For this review, take the finished solid that the model builds, in its own axes (mm). A direction names the side the tool comes from. Round coordinates to 2 decimals unless told otherwise and drop trailing zeros. Loops run counter-clockwise (first coordinate to the right, second up) from the corner with the lowest first, then second, coordinate; pieces in that order, holes last. Notation, with made-up numbers: (85.5, 28) -> (104.5, 28) arc R15 ccw to (104.5, 35) -> close; hole circle Ø3 at (80.5, 89). An arc over 180 degrees is marked (long way). Write each question's results on one line, items separated by ' | '.
```python
from build123d import *

# Parameters (mm, degrees)
SKETCH011_W             = 2000
SKETCH011_H             = 1000
PAD004_DEPTH            = 50
SKETCH012_W             = 100
SKETCH012_H             = 100
PAD005_DEPTH            = 900
SKETCH013_W             = 100
SKETCH013_H             = 100
PAD006_DEPTH            = 900
SKETCH014_W             = 100
SKETCH014_H             = 100
PAD007_DEPTH            = 900
SKETCH015_W             = 100
SKETCH015_H             = 100
PAD008_DEPTH            = 900
FILLET010_R             = 45
BODY002_PLACEMENT_ANGLE = 90


with BuildPart() as part:
    # Sketch011 → Pad004 (new body)
    with BuildSketch(Plane.XY):
        with Locations((1000, 500)):
            Rectangle(SKETCH011_W, SKETCH011_H)
    extrude(amount=PAD004_DEPTH)

    # Sketch012 (on Face5 of Pad004) → Pad005 (join)
    with BuildSketch(Plane(origin=(0, 0, 0), x_dir=(1, 0, 0), z_dir=(0, 0, -1))):
        with Locations((200, -200)):
            Rectangle(SKETCH012_W, SKETCH012_H)
    extrude(amount=PAD005_DEPTH)

    # Sketch013 (on Face4 of Pad005) → Pad006 (join)
    with BuildSketch(Plane(origin=(0, 0, 0), x_dir=(1, 0, 0), z_dir=(0, 0, -1))):
        with Locations((1800, -200)):
            Rectangle(SKETCH013_W, SKETCH013_H)
    extrude(amount=PAD006_DEPTH)

    # Sketch014 (on Face4 of Pad006) → Pad007 (join)
    with BuildSketch(Plane(origin=(0, 0, 0), x_dir=(1, 0, 0), z_dir=(0, 0, -1))):
        with Locations((200, -800)):
            Rectangle(SKETCH014_W, SKETCH014_H)
    extrude(amount=PAD007_DEPTH)

    # Sketch015 (on Face4 of Pad007) → Pad008 (join)
    with BuildSketch(Plane(origin=(0, 0, 0), x_dir=(1, 0, 0), z_dir=(0, 0, -1))):
        with Locations((1800, -800)):
            Rectangle(SKETCH015_W, SKETCH015_H)
    extrude(amount=PAD008_DEPTH)

    # Fillet010
    fillet010_edges = [part.edges().sort_by_distance(p)[0] for p in [
        (1000, 0, 50),
        (2000, 500, 50),
        (1000, 1000, 50),
        (0, 500, 50),
    ]]
    fillet(fillet010_edges, radius=FILLET010_R)


with BuildPart() as part_1:
    # Body002 placement: moved
    add(part.part.moved(Location((2442, 3237, 778))).rotate(Axis((2442, 3237, 778), (0, 0, -1)), BODY002_PLACEMENT_ANGLE))


solid = part_1.part
```
1. For pin 1 (8 mm diameter, centred on x = 2618, z = 599, fed in from +Y), flat-tipped, find the tip position at first contact; note if it passes through.
Values found:
pin 1: stops at y = 3087
2. Consider section A-A (z = 152). State the section outline as (x, y) points, plus the area to 3 significant figures.
Values found:
outline: (2592, 1387) -> (2692, 1387) -> (2692, 1487) -> (2592, 1487) -> close; (2592, 2987) -> (2692, 2987) -> (2692, 3087) -> (2592, 3087) -> close; (3192, 1387) -> (3292, 1387) -> (3292, 1487) -> (3192, 1487) -> close; (3192, 2987) -> (3292, 2987) -> (3292, 3087) -> (3192, 3087) -> close | area: 40,000 mm2
3. Consider section C-C (y = 2106.5). State the section outline as (x, z) points.
Values found:
outline: (2442, 778) -> (3442, 778) -> (3442, 783) arc R45 ccw to (3397, 828) -> (2487, 828) arc R45 ccw to (2442, 783) -> close
4. Draft analysis for pull direction Y (two halves, no side actions). For faces 1 (the face through (2692, 1438, 334)), 2 (the face through (3243, 1487, 334)), 3 (the face through (3243, 3087, 334)), state which applies: released by +Y, released by -Y, zero draft, split by the parting line, or undercut.
Values found:
face 1: zero draft | face 2: undercut | face 3: released by +Y
5. Consider section D-D (x = 3054). State the section outline as (y, z) points.
Values found:
outline: (1237, 778) -> (3237, 778) -> (3237, 783) arc R45 ccw to (3192, 828) -> (1282, 828) arc R45 ccw to (1237, 783) -> close
6. Consider section B-B (x = 2640.5). State the section outline as (y, z) points, plus the area to 3 significant figures.
Values found:
outline: (1237, 778) -> (1387, 778) -> (1387, -122) -> (1487, -122) -> (1487, 778) -> (2987, 778) -> (2987, -122) -> (3087, -122) -> (3087, 778) -> (3237, 778) -> (3237, 783) arc R45 ccw to (3192, 828) -> (1282, 828) arc R45 ccw to (1237, 783) -> close | area: 279,000 mm2
7. To check wall thickness, follow probe 1 along Y at (x, z) = (2688, 122); probe 2 along X at (y, z) = (3033.5, 594); probe 3 along Z at (x, y) = (3152, 2637). State the ranges of each line that lie inside material, in increasing order.
Values found:
probe 1: y = 1387 to 1487, 2987 to 3087 | probe 2: x = 2592 to 2692, 3192 to 3292 | probe 3: z = 778 to 828
8. Tool access review of faces 4 (the face through (2643, 1487, 334)), 5 (the face through (2643, 3087, 334)), 6 (the face through (3192, 3038, 334)), 7 (the face through (2592, 1438, 334)), 8 (the face through (3292, 3038, 334)): name each direction out of +Z, -Z, +X, -X, +Y, -Y from which nothing blocks a thin tool from reaching the whole face with its end or side.
Values found:
face 4: -Z, +X, -X | face 5: -Z, +X, -X, +Y | face 6: -Z, +Y, -Y | face 7: -Z, -X, +Y, -Y | face 8: -Z, +X, +Y, -Y
